from build123d import *

# Parameters (mm, degrees)
F0_W      = 300
F0_H      = 120
F1_DEPTH  = 200
F2_T      = -2.5
F3_W      = 297.5
F3_H      = 197.5
F3_W_2    = 277.5
F3_H_2    = 177.5
F4_DEPTH  = 2.5
F5_R      = 2
F6_DEPTH  = 200.001
F7_R      = 4
F8_DEPTH  = 2.5
F9_R      = 12.5
F10_DEPTH = 25


with BuildPart() as f1:
    # F0 (on Top) → F1 (new body)
    with BuildSketch(Plane.XY):
        with Locations((150, 60)):
            Rectangle(F0_W, F0_H)
    extrude(amount=F1_DEPTH)

    # F2
    f2_openings = [f1.faces().sort_by_distance(p)[0] for p in [
        (150, 120, 100),
    ]]
    offset(amount=F2_T, openings=f2_openings)

    # F3 (on face) → F4 (join)
    with BuildSketch(Plane(origin=(0, 120, 0), x_dir=(-1, 0, 0), z_dir=(0, 1, 0))):
        with Locations((-148.75, 98.75)):
            Rectangle(F3_W, F3_H)
        with Locations((-148.75, 98.75)):
            Rectangle(F3_W_2, F3_H_2, mode=Mode.SUBTRACT)
    extrude(amount=-F4_DEPTH)

    # F5 (on face) → F6 (cut, through all)
    with BuildSketch(Plane.XY.offset(200)):
        with Locations((277.5, 115)):
            Circle(F5_R)
    extrude(amount=-F6_DEPTH, mode=Mode.SUBTRACT)

    # F7 (on face) → F8 (cut)
    with BuildSketch(Plane.XZ):
        with Locations((285, 185)):
            Circle(F7_R)
        with Locations((285, 15)):
            Circle(F7_R)
        with Locations((15, 185)):
            Circle(F7_R)
        with Locations((15, 15)):
            Circle(F7_R)
    extrude(amount=-F8_DEPTH, mode=Mode.SUBTRACT)

    # F9 (on face) → F10 (cut)
    with BuildSketch(Plane.XY):
        with Locations((70, 25)):
            Circle(F9_R)
        with Locations((150, 25)):
            Circle(F9_R)
        with Locations((230, 25)):
            Circle(F9_R)
    extrude(amount=F10_DEPTH, mode=Mode.SUBTRACT)


solid = f1.part
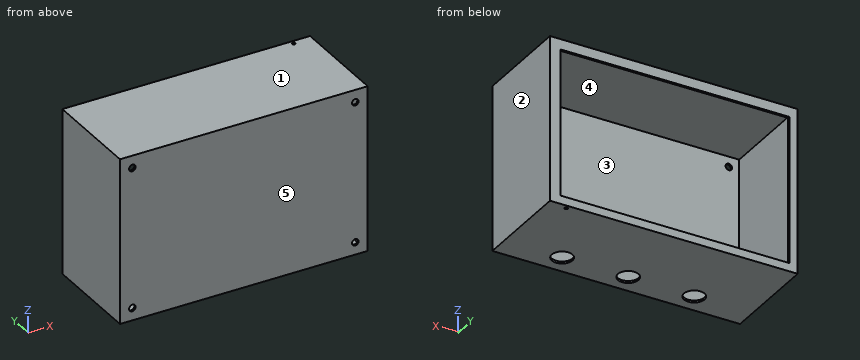
Here's how the part is built. I have some questions about the finished solid (model axes, mm). Face numbers are marked on the shaded views. A direction names the side the tool comes from. Round coordinates to 2 decimals unless told otherwise and drop trailing zeros. Loops run counter-clockwise (first coordinate to the right, second up) from the corner with the lowest first, then second, coordinate; pieces in that order, holes last. Notation, with made-up numbers: M 55,-3 L 102,-3 A26 ccw 102,36 Z; hole C -18,27.5 d5. An arc over 180 degrees is marked long. Write each question's results on one line, items separated by ' | '. Start each with the question number.
(1) If I drill on probe 1 along X at (y, z) = (25, 1.1); probe 2 along Z at (x, y) = (15, 0.85); probe 3 along X at (y, z) = (27.5, 107), over which ranges is the centre line in solid material (lowest first)? Write a range as from..to.
(2) Thinking about a two-plate mould opening in X: for the marked faces 1, 2 and 3, which applies, pulls with the +X half, pulls with the -X half, needs draft (parallel to the pull), parting line crosses it, or undercut?
(3) I want a section at D-D (z = 82.5). Please give me the cut outline in (x, y), then the cut area to 3 significant figures.
(4) On a 3-axis mill with a long thin cutter (end or side, diameter ignored), from which of +Z, -Z, +X, -X, +Y, -Y can I reach the whole of each face in a straight line? I mean the marked faces 4 and 5. Say none if no direction works.
(5) I want a section at A-A (x = 70). Please give me the cut outline in (y, z), then the cut area to 3 significant figures.
(6) I want a section at B-B (z = 15). Please give me the cut outline in (x, y), then the cut area to 3 significant figures.
(7) I want a section at C-C (y = 25). Please give me the cut outline in (x, z).
(8) Will these pins go through, and if not, where does the flat tip stop? P1, Ø3, axis at x = 265.5, z = 175.5, coming from the +Y side; P2, Ø1.5, axis at x = 63, y = 24.5, coming from the -Z side.
Solved:
1) probe 1: x = 0..57.5, 82.5..137.5, 162.5..217.5, 242.5..300 | probe 2: z = 0..11, 19..181, 189..200 | probe 3: x = 0..2.5, 297.5..300
2) face 1: needs draft | face 2: pulls with the +X half | face 3: undercut
3) outline: M 0,0 L 300,0 L 300,120 L 287.5,120 L 287.5,117.5 L 297.5,117.5 L 297.5,2.5 L 2.5,2.5 L 2.5,117.5 L 10,117.5 L 10,120 L 0,120 Z | area: 1,380 mm²
4) face 4: none | face 5: +Z, -Z, +X, -X, -Y
5) outline: M 0,0 L 12.5,0 L 12.5,2.5 L 2.5,2.5 L 2.5,197.5 L 117.5,197.5 L 117.5,187.5 L 120,187.5 L 120,200 L 0,200 Z; M 37.5,0 L 120,0 L 120,10 L 117.5,10 L 117.5,2.5 L 37.5,2.5 Z | area: 1,070 mm²
6) outline: M 0,0 L 11,0 L 11,2.5 L 2.5,2.5 L 2.5,117.5 L 10,117.5 L 10,120 L 0,120 Z; M 19,0 L 281,0 L 281,2.5 L 19,2.5 Z; M 287.5,117.5 L 297.5,117.5 L 297.5,2.5 L 289,2.5 L 289,0 L 300,0 L 300,120 L 287.5,120 Z | area: 1,340 mm²
7) outline: M 0,0 L 57.5,0 L 57.5,2.5 L 2.5,2.5 L 2.5,197.5 L 297.5,197.5 L 297.5,2.5 L 242.5,2.5 L 242.5,0 L 300,0 L 300,200 L 0,200 Z; M 82.5,0 L 137.5,0 L 137.5,2.5 L 82.5,2.5 Z; M 162.5,0 L 217.5,0 L 217.5,2.5 L 162.5,2.5 Z
8) P1: stops at y = 2.5 | P2: stops at z = 197.5
